Work out the finished part from the listing and answer in its coordinate system (mm). Round coordinates to 2 decimals unless told otherwise and drop trailing zeros. Write each loop counter-clockwise with the first axis right and the second up, starting at its lowest first coordinate (ties: lowest second). Pieces come first, ordered by that corner, then holes.
1. Find section B-B (y = -0.4). Count the separate pieces of the cut face and the enclosed holes in it, and give its area (3 significant figures).
2. Flat-ended cylindrical pins translate along their axes: pin 1 Ø3.5 at (x, z) = (-13.04, 16.42) entering from -Y; pin 2 Ø1 at (y, z) = (-0.5, -1.5) entering from +X. Find the tip coordinate at first contact, or state that the pin passes through.
3. Straight lines are drawn through the part: probe 1 along Z at (x, y) = (-12.5, -0.9); probe 2 along X at (y, z) = (-0.2, -7.5); probe 3 along Z at (x, y) = (32, -1.6). For each, find the intervals that lie inside material, in ascending order.
4. Find section A-A (x = -4). Write down the section's boundary in (y, z), and give its area (3 significant figures).
5. Find section C-C (z = 2.5). Write down the section's boundary in (x, y), and give its area (3 significant figures).
6. Find section D-D (x = 31.5). Write down the section's boundary in (y, z), and give its area (3 significant figures).
```python
from build123d import *

# Parameters (mm, degrees)
F0_R     = 2
F1_DEPTH = 2
F2_R     = 2


with BuildPart() as f1:
    # F0 (on Front) → F1 (new body)
    with BuildSketch(Plane.XZ):
        Polygon((-17.038149, 20.423017), (-17.038149, -19.576983), (-9.038149, -19.576983), (-9.038149, 12.423017), (42.961851, 12.423017), (42.961851, 20.423017), align=None)
        with Locations((-13.038149, -13.576983)):
            Circle(F0_R, mode=Mode.SUBTRACT)
        with Locations((-13.038149, -3.576983)):
            Circle(F0_R, mode=Mode.SUBTRACT)
        with Locations((-13.038149, 6.423017)):
            Circle(F0_R, mode=Mode.SUBTRACT)
        with Locations((-13.038149, 16.423017)):
            Circle(F0_R, mode=Mode.SUBTRACT)
        with Locations((-3.038149, 16.423017)):
            Circle(F0_R, mode=Mode.SUBTRACT)
        with Locations((6.961851, 16.423017)):
            Circle(F0_R, mode=Mode.SUBTRACT)
        with Locations((16.961851, 16.423017)):
            Circle(F0_R, mode=Mode.SUBTRACT)
        with Locations((26.961851, 16.423017)):
            Circle(F0_R, mode=Mode.SUBTRACT)
        with Locations((36.961851, 16.423017)):
            Circle(F0_R, mode=Mode.SUBTRACT)
    extrude(amount=F1_DEPTH)

    # F2
    f2_edges = [f1.edges().sort_by_distance(p)[0] for p in [
        (-17.038149, -1, 20.423017),
        (42.961851, -1, 20.423017),
        (42.961851, -1, 12.423017),
        (-9.038149, -1, 12.423017),
        (-9.038149, -1, -19.576983),
        (-17.038149, -1, -19.576983),
    ]]
    fillet(f2_edges, radius=F2_R)


solid = f1.part
```
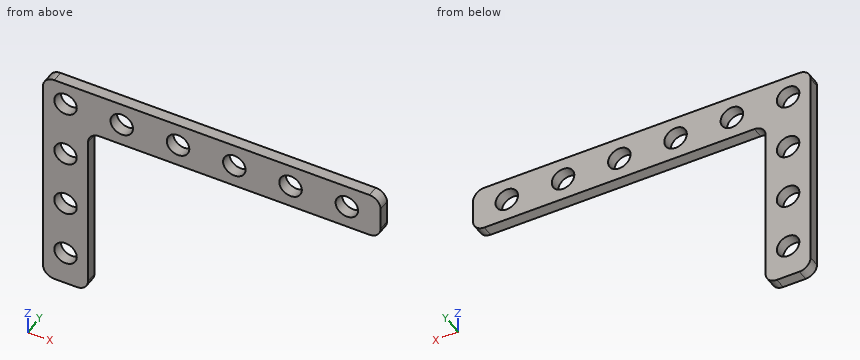
Worked answers:
1. separate pieces: 1
1. enclosed holes: 9
1. area: 619 mm2
2. pin 1: passes through
2. pin 2: stops at x = -9.04
3. probe 1: z = -19.58 to -15.5, -11.65 to -5.5, -1.65 to 4.5, 8.35 to 14.5, 18.35 to 20.42
3. probe 2: x = -17.04 to -9.04
3. probe 3: z = 12.42 to 20.42
4. outline: (-2, 12.42) - (0, 12.42) - (0, 14.67) - (-2, 14.67) - close; (-2, 18.18) - (0, 18.18) - (0, 20.42) - (-2, 20.42) - close
4. area: 8.99 mm2
5. outline: (-17.04, -2) - (-9.04, -2) - (-9.04, 0) - (-17.04, 0) - close
5. area: 16.0 mm2
6. outline: (-2, 12.42) - (0, 12.42) - (0, 20.42) - (-2, 20.42) - close
6. area: 16.0 mm2
